```python
from build123d import *

# Parameters (mm, degrees)
F0_W     = 40
F0_H     = 20
F0_R     = 6.491314
F1_DEPTH = 25
F2_W     = 3
F2_H     = 20
F3_DEPTH = 5
F5_DEPTH = 20.001
F6_R     = 6
F7_DEPTH = 8
F8_R     = 1.258823
F9_DEPTH = 25


with BuildPart() as f1:
    # F0 (on Top) → F1 (new body)
    with BuildSketch(Plane.XY):
        Rectangle(F0_W, F0_H)
        Circle(F0_R, mode=Mode.SUBTRACT)
    extrude(amount=F1_DEPTH)

    # F2 (on face) → F3 (cut)
    with BuildSketch(Plane.XY.offset(25)):
        with Locations((-13.5, 0)):
            Rectangle(F2_W, F2_H)
        with BuildLine():
            Line((2, 10), (-2, 10))
            Line((-2, 10), (-2, 6.175529))
            ThreePointArc((-2, 6.175529), (0, 6.491314), (2, 6.175529))
            Line((2, 6.175529), (2, 10))
        make_face()
        with BuildLine():
            Line((-2, -6.175529), (-2, -10))
            Line((-2, -10), (2, -10))
            Line((2, -10), (2, -6.175529))
            ThreePointArc((2, -6.175529), (0, -6.491314), (-2, -6.175529))
        make_face()
    extrude(amount=-F3_DEPTH, mode=Mode.SUBTRACT)

    # F4 (on face) → F5 (cut, through all)
    with BuildSketch(Plane.XZ.offset(10)):
        Polygon((16, 25), (10, 25), (8.267949, 22), (17.732051, 22), align=None)
    extrude(amount=-F5_DEPTH, mode=Mode.SUBTRACT)

    # F6 (on face) → F7 (join)
    with BuildSketch(Plane.YZ.offset(20)):
        with Locations((0, 12.5)):
            Circle(F6_R)
    extrude(amount=F7_DEPTH)

    # F8 (on face) → F9 (cut)
    with BuildSketch(Plane.YZ.offset(28)):
        with Locations((0, 12.5)):
            Circle(F8_R)
    extrude(amount=-F9_DEPTH, mode=Mode.SUBTRACT)


solid = f1.part
```
Geometry: final body of the model. Coordinates: model frame, mm. A direction names the side the tool comes from. Give positions to 0.01 mm unless a question says otherwise; leave off trailing zeros. Order: outer loops, then holes, each group sorted by start corner. A loop starts at its lowest first (then second) coordinate and runs counter-clockwise, first axis right, second up. Notation, with made-up numbers: M 65.25,88 L 107.25,88 A8 cw 107.25,97 Z; hole C -39.75,-30.5 d9. An arc over 180 degrees is marked long. Answer as CSV lines item,"result". Start each with the question number.
1) Set-up query: faces 1 (the flat face through (20, -2.4, 6.8)), 2 (the flat face through (9.146, -0.14, 23.521)), 3 (the flat face through (0, -10, 12)), 4 (the flat face through (-15, 0, 23)). Return all of +Z, -Z, +X, -X, +Y, -Y with unobstructed straight access to the full face (end or side cutting, diameter ignored); none if empty.
2) Cut plane D-D (z = 6). Output: boundary loops of the cut face in (x, y), then the cut area to 3 significant figures.
3) Cut plane C-C (z = 12.5). Output: boundary loops of the cut face in (x, y).
4) First-contact query: P1, Ø1.5, axis at x = -13, y = 2, coming from the +Z side; P2, Ø4, axis at y = 8, z = 21.5, coming from the +X side. Flat tips, straight axial feed; report the tip coordinate or a pass-through.
5) Mould query, pull axis Y, two halves, no side actions, for faces 5 (the cylindrical face through (23.944, -1.301, 6.643)), 6 (the cylindrical face through (5.996, -2.486, 12.325)), 7 (the flat face through (-2, 8, 23)). Classes: +Y half, -Y half, draft (parallel to the pull), parting line (faces both ways), or undercut.
6) Cut plane B-B (y = 0). Output: boundary loops of the cut face in (x, z), then the cut area to 3 significant figures.
7) Cut plane A-A (x = 0). Output: boundary loops of the cut face in (y, z), then the cut area to 3 significant figures.
8) Line query: line 1 (Y direction, x = 0, z = 15.5); line 2 (X direction, y = -2.25, z = 23); line 3 (Y direction, x = 7, z = 12.5). Output: solid intervals per line, ascending. Write a range as from..to.
Findings below:
1,face 1,"+X"
1,face 2,"+Y, -Y"
1,face 3,"+Z, -Z, +X, -X, -Y"
1,face 4,"+Z, +Y, -Y"
2,outline,"M -20,-10 L 20,-10 L 20,10 L -20,10 Z; hole C 0,0 d12.98"
2,area,"668 mm²"
3,outline,"M -20,-10 L 20,-10 L 20,-6 L 28,-6 L 28,-1.26 L 6.37,-1.26 A6.49 cw long 6.37,1.26 L 28,1.26 L 28,6 L 20,6 L 20,10 L -20,10 Z"
4,P1,"stops at z = 20"
4,P2,"stops at x = 20"
5,face 5,"parting line"
5,face 6,"undercut"
5,face 7,"draft"
6,outline,"M -20,0 L -6.49,0 L -6.49,25 L -12,25 L -12,20 L -15,20 L -15,25 L -20,25 Z; M 6.49,0 L 20,0 L 20,6.5 L 28,6.5 L 28,11.24 L 6.49,11.24 Z; M 6.49,13.76 L 28,13.76 L 28,18.5 L 20,18.5 L 20,25 L 16,25 L 17.73,22 L 8.27,22 L 10,25 L 6.49,25 Z"
6,area,"679 mm²"
7,outline,"M -10,0 L -6.49,0 L -6.49,20 L -10,20 Z; M 6.49,0 L 10,0 L 10,20 L 6.49,20 Z"
7,area,"140 mm²"
8,line 1,"y = -10..-6.49, 6.49..10"
8,line 2,"x = -20..-15, -12..-6.09, 6.09..8.85, 17.15..20"
8,line 3,"y = -10..-1.26, 1.26..10"
